Build history of the part. All positions in model axes, mm. A direction names the side the tool comes from. Coordinates: 2 decimals unless noted, no trailing zeros. Write each loop counter-clockwise with the first axis right and the second up, starting at its lowest first coordinate (ties: lowest second). Pieces come first, ordered by that corner, then holes.
```python
from build123d import *

# Parameters (mm, degrees)
F0_W     = 349.504
F0_H     = 177.8
F1_DEPTH = 19.05
F2_R     = 3.770313
F3_DEPTH = 19.05
F4_R     = 3.770313
F5_DEPTH = 25.4
F6_R     = 4.365625
F7_DEPTH = 25.4
F8_R     = 3.770313
F9_DEPTH = 25.4


with BuildPart() as f1:
    # F0 (on Top) → F1 (new body)
    with BuildSketch(Plane.XY):
        with Locations((174.752, 88.9)):
            Rectangle(F0_W, F0_H)
    extrude(amount=F1_DEPTH)

    # F2 (on face) → F3 (cut)
    with BuildSketch(Plane.YZ.offset(349.504)):
        with Locations((88.9, 9.525)):
            Circle(F2_R)
        with Locations((25.4, 9.525)):
            Circle(F2_R)
        with Locations((152.4, 9.525)):
            Circle(F2_R)
    extrude(amount=-F3_DEPTH, mode=Mode.SUBTRACT)

    # F4 (on face) → F5 (cut)
    with BuildSketch(Plane(origin=(0, 0, 0), x_dir=(0, -1, 0), z_dir=(-1, 0, 0))):
        with Locations((-88.9, 9.525)):
            Circle(F4_R)
        with Locations((-25.4, 9.525)):
            Circle(F4_R)
        with Locations((-152.4, 9.525)):
            Circle(F4_R)
    extrude(amount=-F5_DEPTH, mode=Mode.SUBTRACT)

    # F6 (on face) → F7 (cut)
    with BuildSketch(Plane.XY.offset(19.05)):
        with Locations((98.552, 139.7)):
            Circle(F6_R)
        with Locations((98.552, 38.1)):
            Circle(F6_R)
        with Locations((250.952, 139.7)):
            Circle(F6_R)
        with Locations((250.952, 38.1)):
            Circle(F6_R)
    extrude(amount=-F7_DEPTH, mode=Mode.SUBTRACT)

    # F8 (on face) → F9 (cut)
    with BuildSketch(Plane(origin=(0, 177.8, 0), x_dir=(-1, 0, 0), z_dir=(0, 1, 0))):
        with Locations((-21.844, 9.525)):
            Circle(F8_R)
        with Locations((-65.532, 9.525)):
            Circle(F8_R)
        with Locations((-109.22, 9.525)):
            Circle(F8_R)
        with Locations((-152.908, 9.525)):
            Circle(F8_R)
        with Locations((-196.596, 9.525)):
            Circle(F8_R)
        with Locations((-240.284, 9.525)):
            Circle(F8_R)
        with Locations((-283.972, 9.525)):
            Circle(F8_R)
        with Locations((-327.66, 9.525)):
            Circle(F8_R)
    extrude(amount=-F9_DEPTH, mode=Mode.SUBTRACT)


solid = f1.part
```
1. 3-axis set-ups, long thin cutter, end or side, ignore diameter. For faces 1 (the face through (172, 177.8, 9)), 2 (the face through (12.522, 29.167, 9.691)), 3 (the face through (109, 152.4, 10)): which of +Z, -Z, +X, -X, +Y, -Y reach the whole face in a straight line?
Computed values:
face 1: +Z, -Z, +X, -X, +Y
face 2: -X
face 3: +Y
2. Flat gauge pins, fed straight in: pin 1 (4.5 mm diameter, centred on y = 25.4, z = 9.525, fed in from -X); pin 2 (4 mm diameter, centred on x = 109, z = 10, fed in from +Y); pin 3 (4 mm diameter, centred on y = 88, z = 8.5, fed in from +X); pin 4 (5 mm diameter, centred on x = 250.952, y = 38.1, fed in from -Z). Where does each tip first touch, or does it go through?
Computed values:
pin 1: stops at x = 25.4
pin 2: stops at y = 152.4
pin 3: stops at x = 330.45
pin 4: passes through
3. Mould opens along Y. For faces 4 (the face through (172, 90, 0)), 5 (the face through (66, 152.4, 10)), 6 (the face through (25.4, 25, 10)) say: +Y half, -Y half, draft (parallel to the pull), parting line (faces both ways), or undercut.
Computed values:
face 4: draft
face 5: +Y half
face 6: undercut
4. Saw through at A-A on y = 139.7. List the corners of the cut face in (x, z), plus the area to 3 significant figures.
Computed values:
outline: (0, 0) - (94.19, 0) - (94.19, 19.05) - (0, 19.05) - close; (102.92, 0) - (246.59, 0) - (246.59, 19.05) - (102.92, 19.05) - close; (255.32, 0) - (349.5, 0) - (349.5, 19.05) - (255.32, 19.05) - close
area: 6,330 mm2
5. Probe line 1 along X through (y, z) = (140, 10.25); line 2 along X through (y, z) = (143, 13.5); line 3 along Z through (x, y) = (9.25, 25.4). List the from-to ranges inside material, lowest first.
Computed values:
line 1: x = 0 to 94.2, 102.91 to 246.6, 255.31 to 349.5
line 2: x = 0 to 95.69, 101.41 to 248.09, 253.81 to 349.5
line 3: z = 0 to 5.75, 13.3 to 19.05
